Check sheet for the modelled part. Datum: model origin and axes. Units: mm. A direction names the side the tool comes from. Coordinates: 2 decimals unless noted, no trailing zeros. Order: outer loops, then holes, each group sorted by start corner. A loop starts at its lowest first (then second) coordinate and runs counter-clockwise, first axis right, second up.
Autodesk Inventor part; units mm, degrees
ref_plane "YZ Plane" through (0, 0, 0) normal (1, 0, 0) x (0, 1, 0)
ref_plane "XZ Plane" through (0, 0, 0) normal (0, 1, 0) x (-1, 0, 0)
ref_plane "XY Plane" through (0, 0, 0) normal (0, 0, 1) x (1, 0, 0)
sketch "Sketch1" plane through (0, 0, 0) normal (1, 0, 0) x (0, 1, 0)
  line L0 (0, 0) -> (0, 255)
  line L1 (0, 255) -> (620, 255)
  line L2 (620, 255) -> (620, 265)
  line L3 (-124, 0) -> (744, 0)
  dimension "d0" = 620
  dimension "d1" = 255
  dimension "d2" = 10
surface revolve "RevolutionSrf1" sketch "Sketch1" angle 360 about axis through (0, -10, 0) along (0, 1, 0) shown yes curves L0 L1 L2
thicken "Thicken1" operation new thickness 2 both sides no extend neighbours no toward (0.0589628, 0, -0.9982602) faces at (-15.0355, 413.3333, 254.5563) (258.1049, 620, 5.6577) (70.5152, 0, 40.8296)
properties part number "smietnik1_srodek"
(1) Cross-section at B-B (x = 0). Enter the section's corners in (y, z).
Filled in:
outline: (0, -255) - (620, -255) - (620, -265) - (622, -265) - (622, -253) - (2, -253) - (2, 253) - (622, 253) - (622, 265) - (620, 265) - (620, 255) - (0, 255) - close
(2) Go/stop test with flat-tipped pins: P1, Ø3, axis at x = -41.5, z = -84.5, coming from the -Y side; P2, Ø10, axis at x = 87.5, z = 95, coming from the +Y side; P3, Ø5, axis at x = -57.5, y = 90, coming from the +Z side; P4, Ø1, axis at x = 210.5, y = 432, coming from the -Z side. Record where each tip stops, or that it passes through.
Filled in:
P1: stops at y = 0
P2: stops at y = 2
P3: stops at z = 249
P4: stops at z = -144.65
(3) Cross-section at C-C (y = 416). Enter the section's corners in (x, z), and give its area (3 significant figures).
Filled in:
outline: circle Ø510 at (0, 0); hole circle Ø506 at (0, 0)
area: 3,190 mm2
(4) Thickness scan on probe 1 along X at (y, z) = (450.5, 0); probe 2 along Z at (x, y) = (-5.5, 396); probe 3 along Y at (x, z) = (-65.5, -50.5). Record the ranges inside material, lowest first.
Filled in:
probe 1: x = -255 to -253, 253 to 255
probe 2: z = -254.94 to -252.94, 252.94 to 254.94
probe 3: y = 0 to 2
(5) Release check for a two-part mould opening along X. For faces 3 (the flat face through (4, 2, -4)), 4 (the cylindrical face through (250.847, 316.34, -32.936)), 5 (the flat face through (-97, 622, 234)), 6 (the cylindrical face through (223.45, 621.01, 142.46)) record: +X half, -X half, draft (parallel to the pull), parting line (faces both ways), or undercut.
Filled in:
face 3: undercut
face 4: undercut
face 5: draft
face 6: parting line
(6) Tool access check on faces 1 (the cylindrical face through (-249, 314, -55)), 2 (the flat face through (4, 0, -4)). Record the directions out of +Z, -Z, +X, -X, +Y, -Y that give a thin tool (end or side, any length) a straight path to the whole face; none if there is none.
Filled in:
face 1: -Y
face 2: +Z, -Z, +X, -X, -Y
(7) Cross-section at A-A (z = 0). Enter the section's corners in (x, y).
Filled in:
outline: (-265, 620) - (-255, 620) - (-255, 0) - (255, 0) - (255, 620) - (265, 620) - (265, 622) - (253, 622) - (253, 2) - (-253, 2) - (-253, 622) - (-265, 622) - close
